Check sheet for the modelled part. Datum: model origin and axes. Units: mm. A direction names the side the tool comes from. Give positions to 0.01 mm unless a question says otherwise; leave off trailing zeros. Loops run counter-clockwise (first coordinate to the right, second up) from the corner with the lowest first, then second, coordinate; pieces in that order, holes last. Notation, with made-up numbers: (52, -18) - (66, -18) arc R22 cw to (66, -6) - close; hole circle Ø4 at (33.5, 77.25). An arc over 180 degrees is marked (long way). Answer in a Markdown table with one row per item. Add a question column.
(1) Sectioned sample at A-A on x = 0. Enter the section's corners in (y, z), then the cut area to 4 significant figures.
(2) Draft check along Y on faces 3 (the face through (-6, 0, -1)), 4 (the face through (0, 1.45, 1)), 5 (the face through (0, 0, -2)). Enter one of: released by +Y, released by -Y, zero draft, split by the parting line, or undercut.
(3) Set-up check for faces 1 (the face through (2, -3, 10)), 2 (the face through (-1.262, -0.715, 0.74)): record each of +Z, -Z, +X, -X, +Y, -Y from which the full face is reachable in a straight line by a thin tool's end or side.
(4) Sectioned sample at B-B on z = 6.5. Enter the section's corners in (x, y).
(5) Sectioned sample at D-D on x = 2.25. Enter the section's corners in (y, z).
(6) Sectioned sample at C-C on y = -3. Enter the section's corners in (x, z).
(7) Go/stop test with flat-tipped pins: P1, Ø3, axis at x = 0.5, y = 0.5, coming from the +Z side; P2, Ø5, axis at x = 0.5, z = 7, coming from the -Y side; P3, Ø1, axis at x = -0.5, z = 3, coming from the +Y side. Record where each tip stops, or that it passes through.
(8) Thickness scan on L1, parallel to Y at x = 0, z = 3.75; L2, parallel to Z at x = -5, y = -1.75; L3, parallel to Y at x = 2.25, z = 2. Record the ranges inside material, lowest first.
from build123d import *

# Parameters (mm, degrees)
F0_R     = 6
F0_R_2   = 4.4
F0_R_3   = 3.4
F1_DEPTH = 2
F2_DEPTH = 10
F3_DEPTH = 1.5
F4_DEPTH = 2


with BuildPart() as f1:
    # F0 (on Top) → F1 (new body)
    with BuildSketch(Plane.XY):
        Circle(F0_R)
        Circle(F0_R_2, mode=Mode.SUBTRACT)
        Circle(F0_R_2)
        Circle(F0_R_3, mode=Mode.SUBTRACT)
        Circle(F0_R_3)
        Polygon((0.8371578903, 1.45), (1.6743157806, 0), (0.8371578903, -1.45), (-0.8371578903, -1.45), (-1.6743157806, 0), (-0.8371578903, 1.45), align=None, mode=Mode.SUBTRACT)
    extrude(amount=-F1_DEPTH)

    # F0 (on Top) → F2 (join)
    with BuildSketch(Plane.XY):
        Circle(F0_R_2)
        Circle(F0_R_3, mode=Mode.SUBTRACT)
    extrude(amount=F2_DEPTH)

    # F0 (on Top) → F3 (join)
    with BuildSketch(Plane.XY):
        Polygon((0.8371578903, -1.45), (1.6743157806, 0), (0.8371578903, 1.45), (-0.8371578903, 1.45), (-1.6743157806, 0), (-0.8371578903, -1.45), align=None)
    extrude(amount=F3_DEPTH)

    # F4 (add): a face of the model
    f4_faces = [f1.faces().sort_by_distance(p)[0] for p in [
        (0, 0, 0),
    ]]
    extrude(f4_faces, amount=F4_DEPTH)


solid = f1.part
Reply:
| question | item | result |
|---|---|---|
| 1 | outline | (-6, -2) - (6, -2) - (6, 0) - (4.4, 0) - (4.4, 10) - (3.4, 10) - (3.4, 0) - (1.45, 0) - (1.45, 1.5) - (-1.45, 1.5) - (-1.45, 0) - (-3.4, 0) - (-3.4, 10) - (-4.4, 10) - (-4.4, 0) - (-6, 0) - close |
| 1 | area | 48.35 mm^2 |
| 2 | face 3 | split by the parting line |
| 2 | face 4 | undercut |
| 2 | face 5 | zero draft |
| 3 | face 1 | +Z, +X, -X, +Y, -Y |
| 3 | face 2 | +Z |
| 4 | outline | circle Ø8.8 at (0, 0); hole circle Ø6.8 at (0, 0) |
| 5 | outline | (-5.56, -2) - (5.56, -2) - (5.56, 0) - (3.78, 0) - (3.78, 10) - (2.55, 10) - (2.55, 0) - (-2.55, 0) - (-2.55, 10) - (-3.78, 10) - (-3.78, 0) - (-5.56, 0) - close |
| 6 | outline | (-5.2, -2) - (5.2, -2) - (5.2, 0) - (3.22, 0) - (3.22, 10) - (1.6, 10) - (1.6, 0) - (-1.6, 0) - (-1.6, 10) - (-3.22, 10) - (-3.22, 0) - (-5.2, 0) - close |
| 7 | P1 | z = 1.5 |
| 7 | P2 | y = -4.4 |
| 7 | P3 | y = 4.4 |
| 8 | L1 | -4.4 to -3.4, 3.4 to 4.4 |
| 8 | L2 | -2 to 0 |
| 8 | L3 | -3.78 to -2.55, 2.55 to 3.78 |
